The listing builds one solid part. Answer for the finished solid, in the listing's coordinates (mm). Coordinates: 2 decimals unless noted, no trailing zeros. Order: outer loops, then holes, each group sorted by start corner. A loop starts at its lowest first (then second) coordinate and runs counter-clockwise, first axis right, second up. Notation, with made-up numbers: (12, 30.25) -> (31, 30.25) arc R22 ccw to (31, 55.25) -> close; hole circle Ø4 at (55.25, 5.5). An arc over 180 degrees is marked (long way). Return JSON: item names as keys, results as strings.
Autodesk Inventor part; units mm, degrees
ref_plane "YZ Plane" through (0, 0, 0) normal (1, 0, 0) x (0, 1, 0)
ref_plane "XZ Plane" through (0, 0, 0) normal (0, 1, 0) x (-1, 0, 0)
ref_plane "XY Plane" through (0, 0, 0) normal (0, 0, 1) x (1, 0, 0)
sketch "Sketch1" plane through (0, 0, 0) normal (0, 0, 1) x (1, 0, 0)
  line L0 (-34.925, -57.15) -> (34.925, -57.15)
  line L1 (34.925, -57.15) -> (34.925, 57.15)
  line L2 (34.925, 57.15) -> (-34.925, 57.15)
  line L3 (-34.925, 57.15) -> (-34.925, -57.15)
  line L4 (-34.925, -57.15) -> (34.925, 57.15) construction
  line L5 (34.925, -57.15) -> (-34.925, 57.15) construction
  line L6 (-4.7625, -12.7) -> (4.7625, -12.7)
  line L7 (4.7625, -12.7) -> (4.7625, 12.7)
  line L8 (4.7625, 12.7) -> (-4.7625, 12.7)
  line L9 (-4.7625, 12.7) -> (-4.7625, -12.7)
  line L10 (-4.7625, -12.7) -> (4.7625, 12.7) construction
  line L11 (4.7625, -12.7) -> (-4.7625, 12.7) construction
  point P0 (0, 0)
  dimension "d0" = 69.85
  dimension "d1" = 114.3
  dimension "d2" = 9.525
  dimension "d3" = 25.4
extrude "Extrusion1" add sketch "Sketch1" along normal blind 6
fillet "Fillet1" radius 5.5 4 edges at (0, 57.15, 6) (-34.925, 0, 6) (34.925, 0, 6) (0, -57.15, 6)
sketch "Sketch2" plane through (0, 0, 0) normal (0, 0, -1) x (-1, 0, 0)
  line L0 (-30.925, -53.15) -> (30.925, -53.15)
  line L1 (30.925, -53.15) -> (30.925, 53.15)
  line L2 (30.925, 53.15) -> (-30.925, 53.15)
  line L3 (-30.925, 53.15) -> (-30.925, -53.15)
  line L4 (-30.925, -53.15) -> (30.925, 53.15) construction
  line L5 (30.925, -53.15) -> (-30.925, 53.15) construction
  line L6 (-34.925, 57.15) -> (34.925, 57.15)
  line L7 (34.925, 57.15) -> (34.925, -57.15)
  point P0 (0, 0)
  dimension "d9" = 4
  dimension "d10" = 4
extrude "Extrusion2" cut sketch "Sketch2" against normal blind 4.4
fillet "Fillet2" radius 2 8 edges at (-30.925, 0, 0) (0, -53.15, 0) (0, 53.15, 0) (0, 53.15, 4.4) (30.925, 0, 4.4) (-30.925, 0, 4.4) (30.925, 0, 0) (0, -53.15, 4.4)
sketch "Sketch3" plane through (0, 0, 6) normal (0, 0, 1) x (1, 0, 0)
  circle A0 centre (0, 30.15) radius 2.3813
  circle A1 centre (0, -30.15) radius 2.3813
  point P0 (0, 0)
  dimension "d14" = 60.3
  dimension "d15" = 4.7625
  dimension "d16" = 30.15
  dimension "d18" = 30.15
extrude "Extrusion3" cut sketch "Sketch3" against normal through all
chamfer "Chamfer1" distance 1.6 angle 45 2 edges at (-2.3813, 30.15, 6) (-2.3813, -30.15, 6)
equation "\"d9\" = d10"
properties part number "Light Switch Cover"
1. Determine the mould class of faces 1 (the face through (-6, 1, 4.4)), 2 (the face through (-33.27, -0.8, 4.43)), 3 (the face through (-0.49, 55.5, 4.43)), 4 (the face through (0.49, -55.5, 4.43)) for opening direction Y: pulls with the +Y half, pulls with the -Y half, needs draft (parallel to the pull), parting line crosses it, or undercut.
Answer block:
{"face 1": "undercut", "face 2": "needs draft", "face 3": "pulls with the +Y half", "face 4": "pulls with the -Y half"}
2. The part is cut by section A-A on x = 0. Give the number of separate pieces and of enclosed holes in the cut face, and give its area (3 significant figures).
Answer block:
{"separate pieces": "4", "enclosed holes": "0", "area": "144 mm2"}
3. Each of these flat-tipped pins is pushed along its axis until it touches: pin 1 Ø0.8 at (y, z) = (-6.5, 5.5) entering from -X; pin 2 Ø1.3 at (x, z) = (-1.5, 5) entering from -Y; pin 3 Ø1 at (y, z) = (-40.5, 2.5) entering from -X; pin 4 Ø4.5 at (x, y) = (0, -30.15) entering from +Z. Where does it stop, or does it pass through?
Answer block:
{"pin 1": "stops at x = -32.44", "pin 2": "stops at y = -55.58", "pin 3": "stops at x = -34.72", "pin 4": "passes through"}
4. Consider line 1 (Y direction, x = 0, z = 4.45); line 2 (Z direction, x = 14, y = -49); line 3 (X direction, y = -37, z = 3.25). Determine where each line is inside the solid, lowest interval first. Write a range as from..to.
Answer block:
{"line 1": "y = -55.48..-32.58, -27.72..-12.7, 12.7..27.72, 32.58..55.48", "line 2": "z = 4.4..6", "line 3": "x = -34.19..-30.74, 30.74..34.19"}
5. The part is cut by section C-C on x = 8.5. Give the vertices of the cut face in (y, z).
Answer block:
{"outline": "(-57.15, 0) -> (-55.15, 0) arc R2 ccw to (-53.15, 2) -> (-53.15, 2.4) arc R2 cw to (-51.15, 4.4) -> (51.15, 4.4) arc R2 cw to (53.15, 2.4) -> (53.15, 2) arc R2 ccw to (55.15, 0) -> (57.15, 0) -> (57.15, 0.5) arc R5.5 ccw to (51.65, 6) -> (-51.65, 6) arc R5.5 ccw to (-57.15, 0.5) -> close"}
6. The part is cut by section D-D on y = 22. Give the vertices of the cut face in (x, z) (3 decimals), and give its area (3 significant figures).
Answer block:
{"outline": "(-34.925, 0) -> (-32.925, 0) arc R2 ccw to (-30.925, 2) -> (-30.925, 2.4) arc R2 cw to (-28.925, 4.4) -> (28.925, 4.4) arc R2 cw to (30.925, 2.4) -> (30.925, 2) arc R2 ccw to (32.925, 0) -> (34.925, 0) -> (34.925, 0.5) arc R5.5 ccw to (29.425, 6) -> (-29.425, 6) arc R5.5 ccw to (-34.925, 0.5) -> close", "area": "134 mm2"}
